Could you check a few things on this model? Use its own coordinates, in mm. A direction names the side the tool comes from. Coordinates: 2 decimals unless noted, no trailing zeros. Write each loop counter-clockwise with the first axis right and the second up, starting at its lowest first coordinate (ties: lowest second). Pieces come first, ordered by that corner, then holes. Notation, with made-up numbers: M -7.5,88 L 5.5,88 A30 ccw 5.5,115 Z; hole C 70.25,50 d5. An arc over 180 degrees is marked long. Write item = value, one per line.
```python
from build123d import *

# Parameters (mm, degrees)
BOSS_EXTRUDE1_DEPTH     = 4.7
SKETCH3_R               = 4
SKETCH3_R_2             = 1.5
BOSS_EXTRUDE2_DEPTH     = 17.185
SKETCH4_R               = 5.231012233
BOSS_EXTRUDE3_DEPTH     = 3
CUT_EXTRUDE1_DEPTH      = 24.101519495
CUT_EXTRUDE1_DEPTH_BACK = 24.101519495
SKETCH2_R               = 1.5
CUT_EXTRUDE4_DEPTH      = 2
BOSS_EXTRUDE5_START     = -7
SKETCH7_R               = 5.209530261
SKETCH7_R_2             = 1.5
BOSS_EXTRUDE5_DEPTH     = 2


with BuildPart() as part:
    # Sketch1 → Boss-Extrude1 (new body)
    with BuildSketch(Plane(origin=(0, 0, 0), x_dir=(0, 0, -1), z_dir=(1, 0, 0))):
        Polygon((-4.618711934, -0.028868683), (-2.284354955, -4.014356209), (2.33435698, -3.985487527), (4.618711934, 0.028868683), (2.284354955, 4.014356209), (-2.33435698, 3.985487527), align=None)
    extrude(amount=BOSS_EXTRUDE1_DEPTH)

    # Sketch3 → Boss-Extrude2 (add)
    with BuildSketch(Plane.ZY):
        with Locations(Location((0, 0, 0), (0, 0, 209.641884541))):
            Circle(SKETCH3_R)
        with Locations(Location((0, 0, 0), (0, 0, 180))):
            Circle(SKETCH3_R_2, mode=Mode.SUBTRACT)
    extrude(amount=BOSS_EXTRUDE2_DEPTH)

    # Sketch4 → Boss-Extrude3 (add)
    with BuildSketch(Plane.ZY.offset(17.185)):
        with Locations(Location((0, 0, 0), (0, 0, 270))):
            Circle(SKETCH4_R)
    extrude(amount=-BOSS_EXTRUDE3_DEPTH)

    # Sketch2 → Cut-Extrude1 (cut, two sides: drawn at the far end of the back side and taken through both)
    with BuildSketch(Plane(origin=(4.7, 0, 0), x_dir=(0, 0, -1), z_dir=(1, 0, 0)).offset(-CUT_EXTRUDE1_DEPTH_BACK)):
        Circle(SKETCH2_R)
    extrude(amount=CUT_EXTRUDE1_DEPTH + CUT_EXTRUDE1_DEPTH_BACK, mode=Mode.SUBTRACT)

    # Sketch6 → Cut-Extrude4 (cut)
    with BuildSketch(Plane.ZY.offset(17.185)):
        Polygon((0, -2.886751346), (2.5, -1.443375673), (2.5, 1.443375673), (0, 2.886751346), (-2.5, 1.443375673), (-2.5, -1.443375673), align=None)
    extrude(amount=-CUT_EXTRUDE4_DEPTH, mode=Mode.SUBTRACT)

    # Sketch7 → Boss-Extrude5 (add)
    with BuildSketch(Plane(origin=(0, 0, 0), x_dir=(0, 0, -1), z_dir=(1, 0, 0)).offset(BOSS_EXTRUDE5_START)):
        with Locations(Location((0, 0, 0), (0, 0, 180))):
            Circle(SKETCH7_R)
        Circle(SKETCH7_R_2, mode=Mode.SUBTRACT)
    extrude(amount=BOSS_EXTRUDE5_DEPTH)


solid = part.part
```
Item 1: Imagine slicing it at C-C (y = 4.25). Write out the boundary of the cut face in (x, z) (3 decimals), and give its area (3 significant figures).
Numbers:
outline = M -17.185,-3.05 L -14.185,-3.05 L -14.185,3.05 L -17.185,3.05 Z; M -7,-3.013 L -5,-3.013 L -5,3.013 L -7,3.013 Z
area = 30.3 mm²
Item 2: I'm going to push flat-ended pins straight in: P1, Ø5, axis at x = -1, z = -0.5, coming from the -Y side; P2, Ø1.5, axis at x = -10.5, y = -1, coming from the -Z side; P3, Ø4, axis at y = 0, z = 0, coming from the -X side (3 decimals). Where does each tip first touch, or does it pass through?
Numbers:
P1 = -4.01
P2 = -3.99
P3 = -15.185
Item 3: For faces 1 (the face through (-14.185, -3, -3)), 2 (the face through (0, 3.6, -2.1)), 3 (the face through (2.32, 2.01, 3.46)), 4 (the face through (0, -3.6, -2.1)), which set-ups out of +Z, -Z, +X, -X, +Y, -Y let a thin tool reach every point of the face, with its end or its side?
Numbers:
face_1 = none
face_2 = -Z, +Y
face_3 = +Z, +X, +Y
face_4 = -Z, -Y
Item 4: If I drill on line 1 along Y through (x, z) = (-5.25, 0); line 2 along X through (y, z) = (2.5, 3.25) (3 decimals); line 3 along Z through (x, y) = (-0.5, 0), over which ranges is the centre line in solid material (lowest first)?
Numbers:
line_1 = -5.21 to -1.5, 1.5 to 5.21
line_2 = -17.185 to -14.185, -7 to -5
line_3 = -4 to -1.5, 1.5 to 4
Item 5: Imagine slicing it at A-A (x = 2.5). Write out the boundary of the cut face in (y, z).
Numbers:
outline = M -4.01,2.28 L -3.99,-2.33 L 0.03,-4.62 L 4.01,-2.28 L 3.99,2.33 L -0.03,4.62 Z; hole C 0,0 d3
Item 6: Imagine slicing it at B-B (z = 0.75). Write out the boundary of the cut face in (x, y) (3 decimals).
Numbers:
outline = M -17.185,-5.177 L -14.185,-5.177 L -14.185,-3.929 L -7,-3.929 L -7,-5.155 L -5,-5.155 L -5,-3.929 L 0,-3.929 L 0,-4.005 L 4.7,-4.005 L 4.7,-1.299 L -15.185,-1.299 L -15.185,-2.454 L -17.185,-2.454 Z; M -17.185,2.454 L -15.185,2.454 L -15.185,1.299 L 4.7,1.299 L 4.7,3.995 L 0,3.995 L 0,3.929 L -5,3.929 L -5,5.155 L -7,5.155 L -7,3.929 L -14.185,3.929 L -14.185,5.177 L -17.185,5.177 Z
Item 7: Imagine slicing it at D-D (z = 2). Write out the boundary of the cut face in (x, y) (3 decimals), and give its area (3 significant figures).
Numbers:
outline = M -17.185,-4.834 L -14.185,-4.834 L -14.185,-3.464 L -7,-3.464 L -7,-4.81 L -5,-4.81 L -5,-3.464 L 0,-3.464 L 0,-4.013 L 4.7,-4.013 L 4.7,3.988 L 0,3.988 L 0,3.464 L -5,3.464 L -5,4.81 L -7,4.81 L -7,3.464 L -14.185,3.464 L -14.185,4.834 L -17.185,4.834 L -17.185,1.732 L -15.185,1.732 L -15.185,-1.732 L -17.185,-1.732 Z
area = 163 mm²
Item 8: If we mould it in two halves opening along Y, with no side actions, what happens to faces 5 (the face through (-16.199, 2.175, -1.233)), 6 (the face through (2.32, -2.01, -3.46)), 7 (the face through (-2.465, 3.685, 1.555))? For each: pulls with the +Y half, pulls with the -Y half, needs draft (parallel to the pull), parting line crosses it, or undercut.
Numbers:
face_5 = undercut
face_6 = pulls with the -Y half
face_7 = parting line crosses it
